Input: dimensioned drawing with shaded views. Units: mm. Origin: part minimum x, y, z. A direction names the side the tool comes from. Give positions to 0.01 mm unless a question says otherwise; leave off trailing zeros. Loops run counter-clockwise (first coordinate to the right, second up) from the corner with the lowest first, then second, coordinate; pieces in that order, holes last. Notation, with made-up numbers: M 9.5,33.25 L 29.5,33.25 A19 ccw 29.5,40.25 Z; hole C 59,6 d9. An arc over 180 degrees is marked long. Answer in a Markdown table with one row per item.
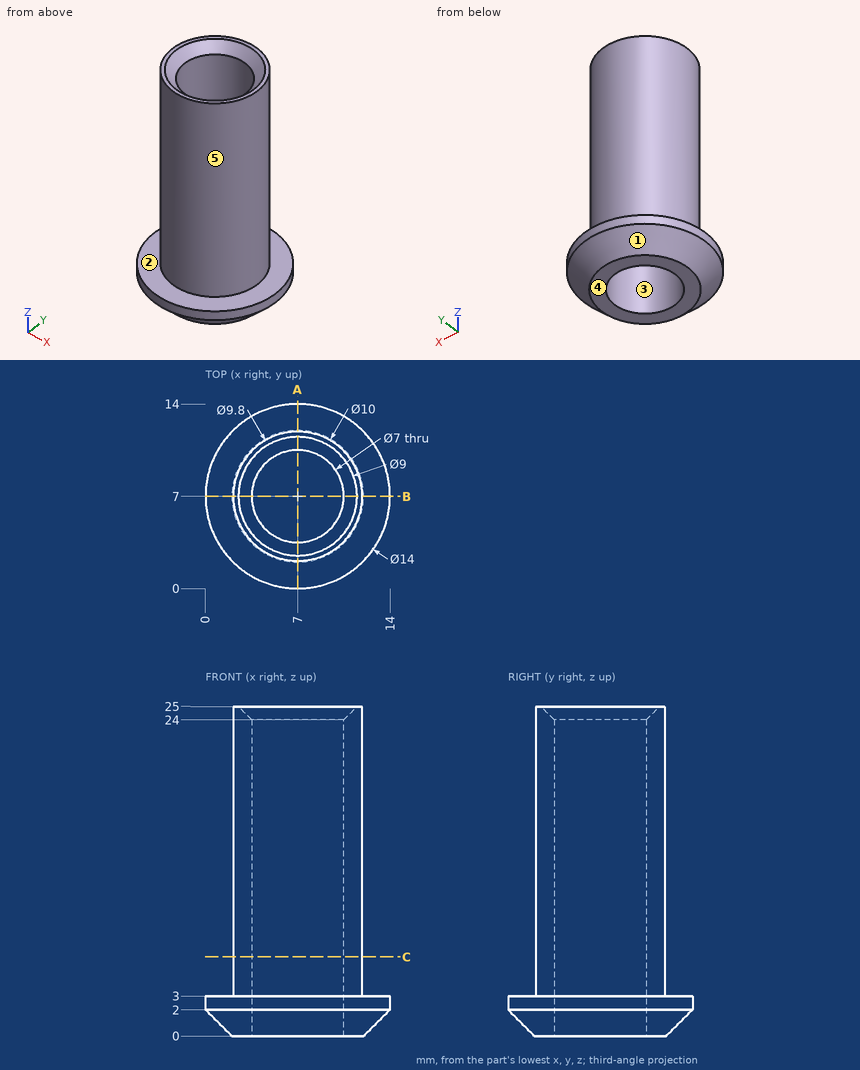
Q1. Section query C-C (z = 6). Output: boundary loops of the cut face in (x, y), plus the area to 3 significant figures.
Values follow:
| item | result |
|---|---|
| outline | C 7,7 d9.8; hole C 7,7 d7 |
| area | 36.9 mm^2 |
Q2. Section query A-A (x = 7). Output: boundary loops of the cut face in (y, z), plus the area to 3 significant figures.
Values follow:
| item | result |
|---|---|
| outline | M 0,2 L 2,0 L 3.5,0 L 3.5,24 L 2.5,25 L 2.1,25 L 2.1,3 L 0,3 Z; M 10.5,0 L 12,0 L 14,2 L 14,3 L 11.9,3 L 11.9,25 L 11.5,25 L 10.5,24 Z |
| area | 77.6 mm^2 |
Q3. Contact query for flat-ended pins moving along their axis: pin 1 Ø2 at (x, z) = (3.5, 14) entering from -Y; pin 2 Ø3 at (y, z) = (8.5, 6) entering from +X; pin 3 Ø8 at (x, z) = (12, 19) entering from -Y. Output: stop coordinate, or through.
Values follow:
| item | result |
|---|---|
| pin 1 | y = 2.79 |
| pin 2 | x = 11.9 |
| pin 3 | y = 2.2 |
Q4. Ray query, probe 1 along Y at (x, z) = (7, 15.25); probe 2 along Y at (x, z) = (5.25, 18.5); probe 3 along X at (y, z) = (9, 5.5). Return the intervals inside material, ascending. Write a range as from..to.
Values follow:
| item | result |
|---|---|
| probe 1 | 2.1..3.5, 10.5..11.9 |
| probe 2 | 2.42..3.97, 10.03..11.58 |
| probe 3 | 2.53..4.13, 9.87..11.47 |
Q5. Reachability of the marked faces 1 and 2 from +Z, -Z, +X, -X, +Y, -Y: full face, straight path, thin tool, end or side. Return the list, or none.
Values follow:
| item | result |
|---|---|
| face 1 | -Z |
| face 2 | +Z |
Q6. Mould query, pull axis X, two halves, no side actions, for the marked faces 3, 4 and 5. Classes: +X half, -X half, draft (parallel to the pull), parting line (faces both ways), or undercut.
Values follow:
| item | result |
|---|---|
| face 3 | undercut |
| face 4 | draft |
| face 5 | parting line |
